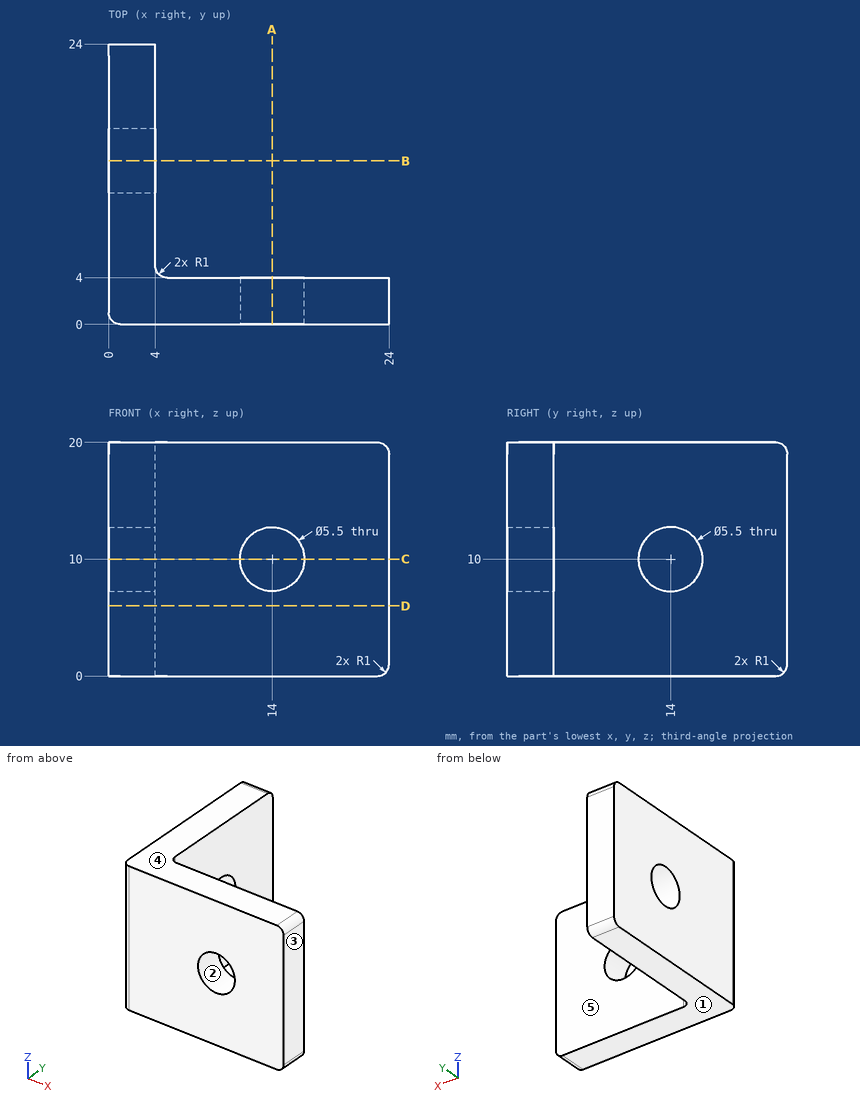
Could you check a few things on this drawing? It's one solid part, dimensions in mm from its lowest x, y, z. A direction names the side the tool comes from. Coordinates: 2 decimals unless noted, no trailing zeros. Loops run counter-clockwise (first coordinate to the right, second up) from the corner with the lowest first, then second, coordinate; pieces in that order, holes last. Notation, with made-up numbers: (-20, 84) - (39, 84) arc R25 ccw to (39, 122) - close; hole circle Ø1 at (0.25, 26.5). An arc over 180 degrees is marked (long way). Return JSON: item names as keys, results as strings. Group by question number.
Item 1: If we section it at D-D on z = 6: Write out the boundary of the cut face in (x, y).
Item 2: On a 3-axis mill with a long thin cutter (end or side, diameter ignored), from which of +Z, -Z, +X, -X, +Y, -Y can I reach the whole of each face in a straight line? I mean the marked faces 4 and 5. Say none if no direction works.
Item 3: Will these pins go through, and if not, where does the flat tip stop? P1, Ø3, axis at x = 6, y = 11, coming from the +Z side; P2, Ø6, axis at y = 8.5, z = 14.5, coming from the +X side.
Item 4: We'd pull the mould along Z, two halves only. Please class the marked faces 1, 2 and 3: +Z half, -Z half, draft (parallel to the pull), parting line (faces both ways), or undercut.
Item 5: I need wall thicknesses on line 1 (Z direction, x = 2.65, y = 14); line 2 (X direction, y = 7, z = 17.75). Which ranges of each line are inside material? Lowest first, please. Write a range as from..to.
Item 6: If we section it at A-A on x = 14: Write out the boundary of the cut face in (y, z).
Item 7: If we section it at C-C on z = 10: Write out the boundary of the cut face in (x, y).
Calculated:
{
 "1": {"outline": "(0, 1) arc R1 ccw to (1, 0) - (24, 0) - (24, 4) - (5, 4) arc R1 cw to (4, 5) - (4, 24) - (0, 24) - close"},
 "2": {"face 4": "+Z, +X, -X, +Y, -Y", "face 5": "+Z, -Z, +X, +Y"},
 "3": {"P1": "passes through", "P2": "stops at x = 4"},
 "4": {"face 1": "-Z half", "face 2": "undercut", "face 3": "draft"},
 "5": {"line 1": "z = 0..7.25, 12.75..20", "line 2": "x = 0..4"},
 "6": {"outline": "(0, 0) - (4, 0) - (4, 7.25) - (0, 7.25) - close; (0, 12.75) - (4, 12.75) - (4, 20) - (0, 20) - close"},
 "7": {"outline": "(0, 1) arc R1 ccw to (1, 0) - (11.25, 0) - (11.25, 4) - (5, 4) arc R1 cw to (4, 5) - (4, 11.25) - (0, 11.25) - close; (0, 16.75) - (4, 16.75) - (4, 24) - (0, 24) - close; (16.75, 0) - (24, 0) - (24, 4) - (16.75, 4) - close"}
}
